Geometry: final body of the model. Coordinates: model frame, mm. Face numbers are marked on the shaded views. A direction names the side the tool comes from. Give positions to 0.01 mm unless a question says otherwise; leave off trailing zeros. Write each loop counter-clockwise with the first axis right and the second up, starting at its lowest first coordinate (ties: lowest second). Pieces come first, ordered by that corner, then holes.
Q1. Line query: L1, parallel to Z at x = -12.7, y = 2.5; L2, parallel to Z at x = 12.7, y = 4.25; L3, parallel to X at y = 9.5, z = 22. Output: solid intervals per line, ascending.
Q2. Cut plane A-A on x = 12.7. Return the cut outline in (y, z).
Q3. Reachability of the marked faces 4, 5, 6, 7 and 8 from +Z, -Z, +X, -X, +Y, -Y: full face, straight path, thin tool, end or side. Return the list, or none.
Q4. Pin query (flat end, axial travel): pin 1 (3.5 mm diameter, centred on x = -13.5, z = 21.5, fed in from +Y); pin 2 (6 mm diameter, centred on x = 12.7, z = -19.05, fed in from -Y); pin 3 (2 mm diameter, centred on y = 5, z = 11.5, fed in from +X); pin 4 (5 mm diameter, centred on y = 2, z = -5, fed in from -X). Return the tip coordinate at first contact, or that it passes through.
Q5. Cut plane B-B on z = -19.05. Return the cut outline in (x, y).
Q6. Cut plane D-D on x = -2. Return the cut outline in (y, z), plus the area to 3 significant figures.
Q7. Cut plane C-C on y = 10.25. Return the cut outline in (x, z), plus the area to 3 significant figures.
Q8. Draft query along Z for the marked faces 1, 2 and 3. Return one class per face: pulls with the +Z half, pulls with the -Z half, needs draft (parallel to the pull), parting line crosses it, or undercut.
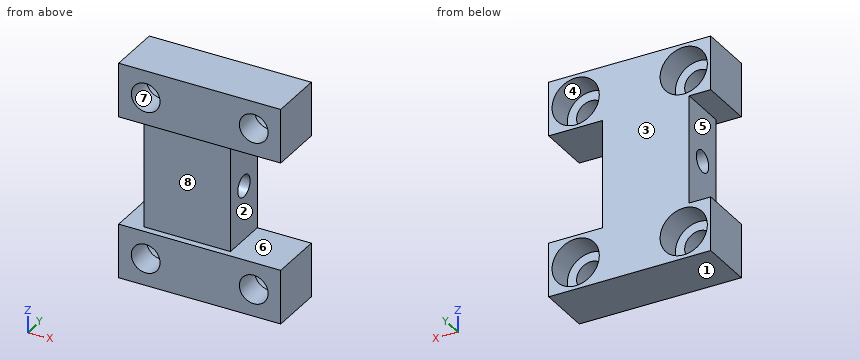
```python
from build123d import *

# Parameters (mm, degrees)
SKETCH1_W                                        = 38.1
SKETCH1_H                                        = 50.8
EXTRUDE1_DEPTH                                   = 12.7
CBORE_FOR_1_4_SOCKET_HEAD_CAP_SCREW1_D           = 6.7564
CBORE_FOR_1_4_SOCKET_HEAD_CAP_SCREW1_CBORE_D     = 11.1125
CBORE_FOR_1_4_SOCKET_HEAD_CAP_SCREW1_CBORE_DEPTH = 6.35
SKETCH3_W                                        = 5.08
SKETCH3_H                                        = 25.4
SKETCH3_W_2                                      = 12.7
CUT_EXTRUDE2_DEPTH                               = 35.195796525
SKETCH5_W                                        = 20.32
SKETCH5_H                                        = 25.4
CUT_EXTRUDE4_DEPTH                               = 1.5875
F_1_4_20_TAPPED_HOLE1_D                          = 5.1054


with BuildPart() as part:
    # Sketch1 → Extrude1 (new body)
    with BuildSketch(Plane(origin=(0, 0, 0), x_dir=(1, 0, 0), z_dir=(0, 1, 0))):
        Rectangle(SKETCH1_W, SKETCH1_H)
    extrude(amount=EXTRUDE1_DEPTH)

    # CBORE for 1/4 Socket Head Cap Screw1 (through all)
    with Locations(Plane(origin=(0, 12.7, 0), x_dir=(-1, 0, 0), z_dir=(0, 1, 0))):
        with Locations((12.7, -19.05), (-12.7, -19.05), (-12.7, 19.05), (12.7, 19.05)):
            CounterBoreHole(CBORE_FOR_1_4_SOCKET_HEAD_CAP_SCREW1_D / 2, CBORE_FOR_1_4_SOCKET_HEAD_CAP_SCREW1_CBORE_D / 2, CBORE_FOR_1_4_SOCKET_HEAD_CAP_SCREW1_CBORE_DEPTH)

    # Sketch3 → Cut-Extrude2 (cut, through all)
    with BuildSketch(Plane(origin=(0, 12.7, 0), x_dir=(-1, 0, 0), z_dir=(0, 1, 0))):
        with Locations((16.51, 0)):
            Rectangle(SKETCH3_W, SKETCH3_H)
        with Locations((-12.7, 0)):
            Rectangle(SKETCH3_W_2, SKETCH3_H)
    extrude(amount=-CUT_EXTRUDE2_DEPTH, mode=Mode.SUBTRACT)

    # Sketch5 → Cut-Extrude4 (cut)
    with BuildSketch(Plane.XZ):
        with Locations((-3.81, 0)):
            Rectangle(SKETCH5_W, SKETCH5_H)
    extrude(amount=-CUT_EXTRUDE4_DEPTH, mode=Mode.SUBTRACT)

    # 1/4-20 Tapped Hole1 (through all)
    with Locations(Plane.ZY.offset(13.97)):
        with Locations((0, 7.14375)):
            Hole(F_1_4_20_TAPPED_HOLE1_D / 2)


solid = part.part
```
Data:
1. L1: z = -25.4 to -22.43, -15.67 to 15.67, 22.43 to 25.4
1. L2: z = -25.4 to -22.43, -15.67 to -12.7, 12.7 to 15.67, 22.43 to 25.4
1. L3: x = -19.05 to -17.41, -7.99 to 7.99, 17.41 to 19.05
2. outline: (0, -25.4) - (12.7, -25.4) - (12.7, -24.61) - (6.35, -24.61) - (6.35, -22.43) - (0, -22.43) - close; (0, -15.67) - (6.35, -15.67) - (6.35, -13.49) - (12.7, -13.49) - (12.7, -12.7) - (0, -12.7) - close; (0, 12.7) - (12.7, 12.7) - (12.7, 13.49) - (6.35, 13.49) - (6.35, 15.67) - (0, 15.67) - close; (0, 22.43) - (6.35, 22.43) - (6.35, 24.61) - (12.7, 24.61) - (12.7, 25.4) - (0, 25.4) - close
3. face 4: +Y
3. face 5: -X, +Y, -Y
3. face 6: -Y
3. face 7: +Y, -Y
3. face 8: +X, -X, -Y
4. pin 1: stops at y = 6.35
4. pin 2: passes through
4. pin 3: stops at x = 6.35
4. pin 4: stops at x = -13.97
5. outline: (-19.05, 0) - (-16.08, 0) - (-16.08, 6.35) - (-18.26, 6.35) - (-18.26, 12.7) - (-19.05, 12.7) - close; (-9.32, 0) - (9.32, 0) - (9.32, 6.35) - (7.14, 6.35) - (7.14, 12.7) - (-7.14, 12.7) - (-7.14, 6.35) - (-9.32, 6.35) - close; (16.08, 0) - (19.05, 0) - (19.05, 12.7) - (18.26, 12.7) - (18.26, 6.35) - (16.08, 6.35) - close
6. outline: (0, -25.4) - (12.7, -25.4) - (12.7, 25.4) - (0, 25.4) - (0, 12.7) - (1.59, 12.7) - (1.59, -12.7) - (0, -12.7) - close; hole circle Ø5.11 at (7.14, 0)
6. area: 584 mm2
7. outline: (-19.05, -25.4) - (19.05, -25.4) - (19.05, -12.7) - (6.35, -12.7) - (6.35, 12.7) - (19.05, 12.7) - (19.05, 25.4) - (-19.05, 25.4) - (-19.05, 12.7) - (-13.97, 12.7) - (-13.97, -12.7) - (-19.05, -12.7) - close; hole circle Ø11.11 at (-12.7, -19.05); hole circle Ø11.11 at (-12.7, 19.05); hole circle Ø11.11 at (12.7, -19.05); hole circle Ø11.11 at (12.7, 19.05)
7. area: 1,100 mm2
8. face 1: pulls with the -Z half
8. face 2: undercut
8. face 3: needs draft
